from build123d import *

# Parameters (mm, degrees)
SKETCH1_W                = 203.2
SKETCH1_H                = 139.7
BASE_EXTRUDE_DEPTH       = 0.127
SKETCH2_W                = 152.4
SKETCH2_H                = 88.9
CENTER_CUT_DEPTH         = 124.294763186
SKETCH3_W                = 38.1
SKETCH3_H                = 215.9
VETICAL_CUT_DEPTH        = 124.294763186
FILLET_1_R               = 31.75
SKETCH4_W                = 6.35
SKETCH4_H                = 6.35
SQUARE_EXTRUDE_DEPTH     = 0.127
SKETCH7_R                = 3.3782
CIRCULAR_EXTRUDE_DEPTH   = 124.294763186
MIRROR_2_COPY_1_SKETCH_R = 3.3782
MIRROR_2_COPY_1_DEPTH    = 124.294763186
FILLET_2_R               = 6.35


with BuildPart() as part:
    # Sketch1 → Base Extrude (new body)
    with BuildSketch(Plane(origin=(0, 0, 0), x_dir=(1, 0, 0), z_dir=(0, 1, 0))):
        Rectangle(SKETCH1_W, SKETCH1_H)
    extrude(amount=BASE_EXTRUDE_DEPTH)

    # Sketch2 → Center Cut (cut, through all)
    with BuildSketch(Plane(origin=(0, 0.127, 0), x_dir=(1, 0, 0), z_dir=(0, 1, 0))):
        Rectangle(SKETCH2_W, SKETCH2_H)
    extrude(amount=-CENTER_CUT_DEPTH, mode=Mode.SUBTRACT)

    # Sketch3 → Vetical Cut (cut, through all)
    with BuildSketch(Plane(origin=(0, 0.127, 0), x_dir=(1, 0, 0), z_dir=(0, 1, 0))):
        with Locations((0, -44.45)):
            Rectangle(SKETCH3_W, SKETCH3_H)
    extrude(amount=-VETICAL_CUT_DEPTH, mode=Mode.SUBTRACT)

    # Fillet 1
    fillet_1_edges = [part.edges().sort_by_distance(p)[0] for p in [
        (-101.6, 0.0635, -69.85),
        (101.6, 0.0635, -69.85),
        (101.6, 0.0635, 69.85),
        (-101.6, 0.0635, 69.85),
    ]]
    fillet(fillet_1_edges, radius=FILLET_1_R)

    # Sketch4 → Square Extrude (add)
    with BuildSketch(Plane(origin=(0, 0.127, 0), x_dir=(1, 0, 0), z_dir=(0, 1, 0))):
        with Locations((-19.05, -61.595)):
            Rectangle(SKETCH4_W, SKETCH4_H)
    extrude(amount=-SQUARE_EXTRUDE_DEPTH)

    # Sketch7 → Circular Extrude (cut, through all)
    with BuildSketch(Plane(origin=(0, 0.127, 0), x_dir=(1, 0, 0), z_dir=(0, 1, 0))):
        with Locations(Location((-93.345, -19.05, 0), (0, 0, 270))):
            Circle(SKETCH7_R)
        with Locations(Location((-86.463473824, -54.713473824, 0), (0, 0, 270))):
            Circle(SKETCH7_R)
        with Locations(Location((-30.48, -61.595, 0), (0, 0, 270))):
            Circle(SKETCH7_R)
        with Locations(Location((-54.61, -61.595, 0), (0, 0, 270))):
            Circle(SKETCH7_R)
    circular_extrude = extrude(amount=-CIRCULAR_EXTRUDE_DEPTH, mode=Mode.SUBTRACT)

    # Mirror 1: Circular Extrude across plane
    add(circular_extrude.mirror(Plane(origin=(0, 0, 0), x_dir=(0, 0, 1), z_dir=(1, 0, 0))), mode=Mode.SUBTRACT)

    # Mirror 2: Circular Extrude across plane
    add(circular_extrude.mirror(Plane.XY), mode=Mode.SUBTRACT)

    # Mirror 2 copy 1 sketch → Mirror 2 copy 1 (cut, through all)
    with BuildSketch(Plane(origin=(0, 0.127, 0), x_dir=(-1, 0, 0), z_dir=(0, 1, 0))):
        with Locations(Location((-93.345, -19.05, 0), (0, 0, 270))):
            Circle(MIRROR_2_COPY_1_SKETCH_R)
        with Locations(Location((-86.463473824, -54.713473824, 0), (0, 0, 270))):
            Circle(MIRROR_2_COPY_1_SKETCH_R)
        with Locations(Location((-30.48, -61.595, 0), (0, 0, 270))):
            Circle(MIRROR_2_COPY_1_SKETCH_R)
        with Locations(Location((-54.61, -61.595, 0), (0, 0, 270))):
            Circle(MIRROR_2_COPY_1_SKETCH_R)
    extrude(amount=-MIRROR_2_COPY_1_DEPTH, mode=Mode.SUBTRACT)

    # Fillet 2
    fillet_2_edges = [part.edges().sort_by_distance(p)[0] for p in [
        (-76.2, 0.0635, 44.45),
        (-76.2, 0.0635, -44.45),
        (76.2, 0.0635, -44.45),
        (76.2, 0.0635, 44.45),
    ]]
    fillet(fillet_2_edges, radius=FILLET_2_R)


solid = part.part
Read the model definition and answer for the solid it produces. Units are mm, in the model's axes. Round coordinates to 2 decimals unless told otherwise and drop trailing zeros. Write each loop counter-clockwise with the first axis right and the second up, starting at its lowest first coordinate (ties: lowest second). Pieces come first, ordered by that corner, then holes.
1. The part is cut by section A-A, the plane x = 54.61. Determine the outline of the cut face in (y, z).
2. Given pin 1 Ø6 at (x, z) = (30.48, 61.595) entering from -Y, flat-ended and moving along its own axis, determine where the tip first touches the part or whether it passes through.
3. The part is cut by section D-D, the plane y = 0.05. State how many separate pieces and enclosed holes the cut face has, then the cut area to 3 significant figures.
4. The part is cut by section C-C, the plane x = -61.5. Determine the outline of the cut face in (y, z).
5. Straight lines are drawn through the part: L1, parallel to Z at x = 47, y = 0.05; L2, parallel to X at y = 0.05, z = -25. For each, find the intervals that lie inside material, in ascending order.
6. The part is cut by section B-B, the plane z = -19.05. Determine the outline of the cut face in (x, y), then the cut area to 3 significant figures.
Values:
1. outline: (0, -69.85) - (0.13, -69.85) - (0.13, -64.97) - (0, -64.97) - close; (0, -58.22) - (0.13, -58.22) - (0.13, -44.45) - (0, -44.45) - close; (0, 44.45) - (0.13, 44.45) - (0.13, 58.22) - (0, 58.22) - close; (0, 64.97) - (0.13, 64.97) - (0.13, 69.85) - (0, 69.85) - close
2. pin 1: passes through
3. separate pieces: 1
3. enclosed holes: 16
3. area: 11,800 mm2
4. outline: (0, -69.85) - (0.13, -69.85) - (0.13, -44.45) - (0, -44.45) - close; (0, 44.45) - (0.13, 44.45) - (0.13, 69.85) - (0, 69.85) - close
5. L1: z = -69.85 to -44.45, 44.45 to 69.85
5. L2: x = -101.6 to -76.2, 76.2 to 101.6
6. outline: (-101.6, 0) - (-96.72, 0) - (-96.72, 0.13) - (-101.6, 0.13) - close; (-89.97, 0) - (-76.2, 0) - (-76.2, 0.13) - (-89.97, 0.13) - close; (76.2, 0) - (89.97, 0) - (89.97, 0.13) - (76.2, 0.13) - close; (96.72, 0) - (101.6, 0) - (101.6, 0.13) - (96.72, 0.13) - close
6. area: 4.74 mm2
